Could you check a few things on this drawing? It's one solid part, dimensions in mm from its lowest x, y, z. A direction names the side the tool comes from. Round coordinates to 2 decimals unless told otherwise and drop trailing zeros. Order: outer loops, then holes, each group sorted by start corner. A loop starts at its lowest first (then second) coordinate and runs counter-clockwise, first axis right, second up.
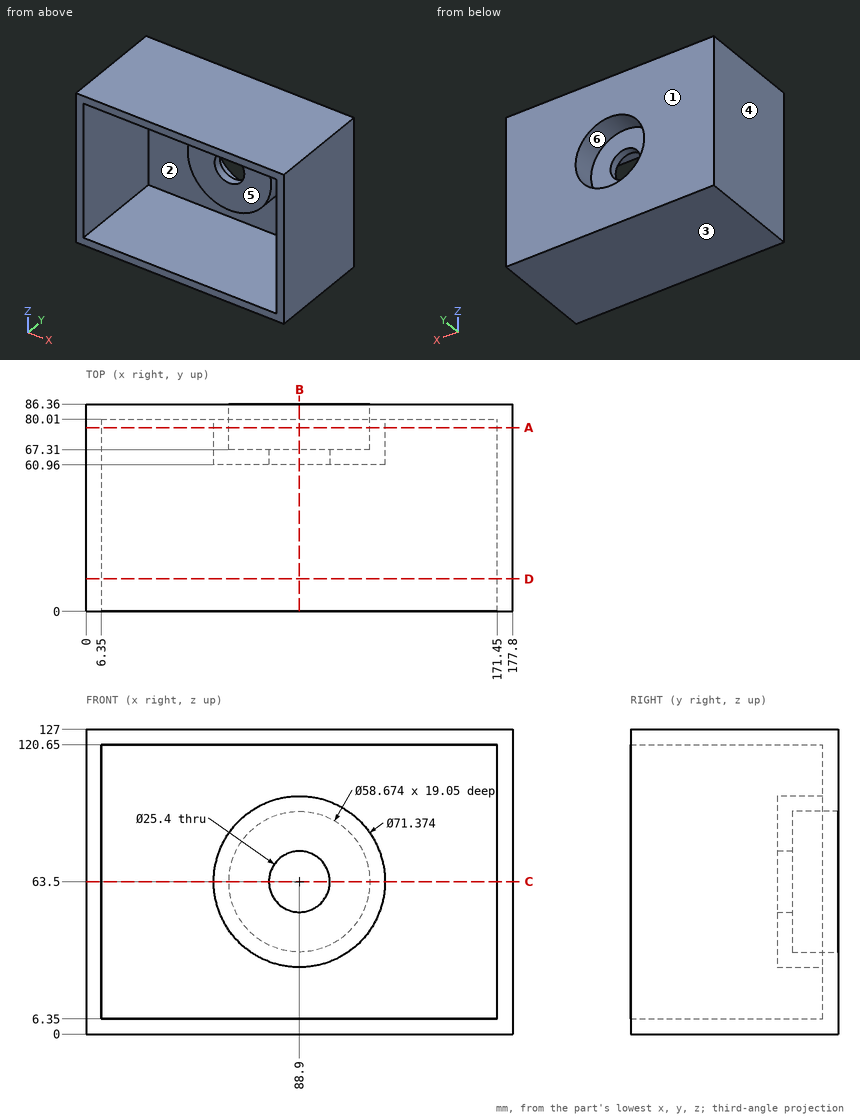
(1) Please list where these lines run through material, in increasing order: probe 1 along X at (y, z) = (65, 63.5); probe 2 along Z at (x, y) = (88, 75); probe 3 along X at (y, z) = (27.5, 112).
(2) I'm going to push flat-ended pins straight in: pin 1 Ø10 at (x, z) = (51, 27.5) entering from -Y; pin 2 Ø2 at (x, z) = (104.5, 61.5) entering from -Y; pin 3 Ø12 at (y, z) = (32, 35.5) entering from -X. Where does each tip first touch, or does it pass through?
(3) I want a section at D-D, the plane y = 13.5. List the corners of the cut face in (x, z) for me.
(4) If we mould it in two halves opening along Z, with no side actions, what happens to the marked faces 1, 2 and 3? For each: pulls with the +Z half, pulls with the -Z half, needs draft (parallel to the pull), parting line crosses it, or undercut.
(5) I want a section at C-C, the plane z = 63.5. List the corners of the cut face in (x, y) for me, plus the area to 3 significant figures.
(6) I want a section at B-B, the plane x = 88.9. List the corners of the cut face in (y, z) for me.
(7) I want a section at A-A, the plane y = 76.5. List the corners of the cut face in (x, z) for me.
(8) On a 3-axis mill with a long thin cutter (end or side, diameter ignored), from which of +Z, -Z, +X, -X, +Y, -Y can I reach the whole of each face in a straight line? I mean the marked faces 4, 5 and 6. Say none if no direction works.
Ans:
1. probe 1: x = 0 to 6.35, 53.21 to 76.2, 101.6 to 124.59, 171.45 to 177.8
1. probe 2: z = 0 to 6.35, 27.82 to 34.18, 92.82 to 99.18, 120.65 to 127
1. probe 3: x = 0 to 6.35, 171.45 to 177.8
2. pin 1: stops at y = 80.01
2. pin 2: stops at y = 60.96
2. pin 3: stops at x = 0
3. outline: (0, 0) - (177.8, 0) - (177.8, 127) - (0, 127) - close; hole (6.35, 6.35) - (171.45, 6.35) - (171.45, 120.65) - (6.35, 120.65) - close
4. face 1: needs draft
4. face 2: undercut
4. face 3: pulls with the -Z half
5. outline: (0, 0) - (6.35, 0) - (6.35, 80.01) - (53.21, 80.01) - (53.21, 60.96) - (76.2, 60.96) - (76.2, 67.31) - (59.56, 67.31) - (59.56, 86.36) - (0, 86.36) - close; (101.6, 60.96) - (124.59, 60.96) - (124.59, 80.01) - (171.45, 80.01) - (171.45, 0) - (177.8, 0) - (177.8, 86.36) - (118.24, 86.36) - (118.24, 67.31) - (101.6, 67.31) - close
5. area: 2,230 mm2
6. outline: (0, 0) - (86.36, 0) - (86.36, 34.16) - (67.31, 34.16) - (67.31, 50.8) - (60.96, 50.8) - (60.96, 27.81) - (80.01, 27.81) - (80.01, 6.35) - (0, 6.35) - close; (0, 120.65) - (80.01, 120.65) - (80.01, 99.19) - (60.96, 99.19) - (60.96, 76.2) - (67.31, 76.2) - (67.31, 92.84) - (86.36, 92.84) - (86.36, 127) - (0, 127) - close
7. outline: (0, 0) - (177.8, 0) - (177.8, 127) - (0, 127) - close; circle Ø71.37 at (88.9, 63.5); hole (6.35, 6.35) - (171.45, 6.35) - (171.45, 120.65) - (6.35, 120.65) - close; hole circle Ø58.67 at (88.9, 63.5)
8. face 4: +Z, -Z, -X, +Y, -Y
8. face 5: -Y
8. face 6: +Y
